Verification items for the finished model (mm, model axes). Coordinates: 2 decimals unless noted, no trailing zeros. Order: outer loops, then holes, each group sorted by start corner. A loop starts at its lowest first (then second) coordinate and runs counter-clockwise, first axis right, second up.
Q1. Cross-section at B-B, the plane z = 0. Record the boundary of the cut face in (x, y), and give its area (3 significant figures).
Q2. Cross-section at C-C, the plane y = -4.5. Count the separate pieces of the cut face and the enclosed holes in it, and give its area (3 significant figures).
Q3. Cross-section at D-D, the plane z = 36. Record the boundary of the cut face in (x, y).
Q4. Depth check by flat-ended pin: P1, Ø8.5, axis at x = 70.71, z = 70.71, coming from the -Y side; P2, Ø3.5, axis at x = -7.5, z = 0, coming from the +Y side; P3, Ø3, axis at y = -2.5, z = 75.5, coming from the -X side; P4, Ø2, axis at x = 6.5, y = -4.5, coming from the -Z side. Enter the tip coordinate at first touch or a pass-through.
Q5. Thickness scan on line 1 (X direction, y = -3.45, z = 0); line 2 (X direction, y = -2.65, z = 7.5); line 3 (Z direction, x = 69.5, y = -3.25). Record the ranges inside material, lowest first.
Q6. Cross-section at A-A, the plane x = 7.5. Record the boundary of the cut face in (y, z), and give its area (3 significant figures).
from build123d import *

# Parameters (mm, degrees)
SKETCH2_R                                       = 4.7625
SKETCH2_W                                       = 6.1
SKETCH2_H                                       = 6.1
BOSS_EXTRUDE1_DEPTH                             = 6.35
CSK_FOR_M3_FLAT_HEAD_MACHINE_SCREW1_D           = 3.2
CSK_FOR_M3_FLAT_HEAD_MACHINE_SCREW1_CSINK_D     = 6.3
CSK_FOR_M3_FLAT_HEAD_MACHINE_SCREW1_CSINK_ANGLE = 90


with BuildPart() as part:
    # Sketch2 → Boss-Extrude1 (new body)
    with BuildSketch(Plane(origin=(0, 0, 0), x_dir=(1, 0, 0), z_dir=(0, 1, 0))):
        with BuildLine():
            Line((10.606601718, 10.606601718), (81.317279836, -60.104076401))
            ThreePointArc((81.317279836, -60.104076401), (81.317279836, -81.317279836), (60.104076401, -81.317279836))
            Line((60.104076401, -81.317279836), (-10.606601718, -10.606601718))
            ThreePointArc((-10.606601718, -10.606601718), (-10.606601718, 10.606601718), (10.606601718, 10.606601718))
        make_face()
        with Locations(Location((70.710678119, -70.710678119, 0), (0, 0, 270))):
            Circle(SKETCH2_R, mode=Mode.SUBTRACT)
        Rectangle(SKETCH2_W, SKETCH2_H, mode=Mode.SUBTRACT)
    extrude(amount=-BOSS_EXTRUDE1_DEPTH)

    # CSK for M3 Flat Head Machine Screw1 (through all)
    with Locations(Plane(origin=(0, 0, -7.5), x_dir=(0, 0, 1), z_dir=(0, 1, 0))):
        with Locations((0, 0), (7.5, -7.5), (7.5, 7.5), (15, 0)):
            CounterSinkHole(CSK_FOR_M3_FLAT_HEAD_MACHINE_SCREW1_D / 2, CSK_FOR_M3_FLAT_HEAD_MACHINE_SCREW1_CSINK_D / 2, counter_sink_angle=CSK_FOR_M3_FLAT_HEAD_MACHINE_SCREW1_CSINK_ANGLE)


solid = part.part
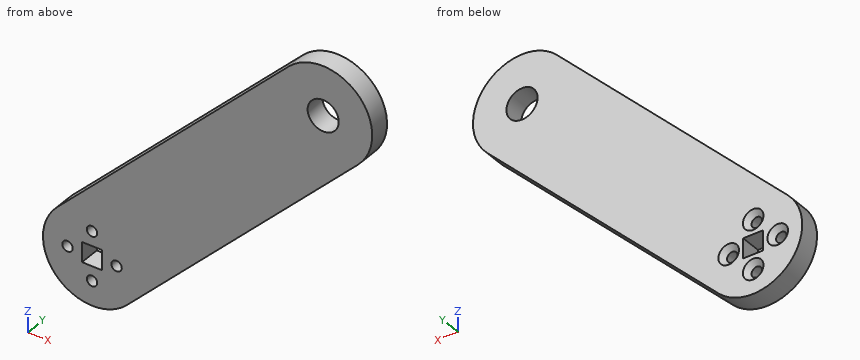
Check values:
1. outline: (-15, -6.35) - (-9.1, -6.35) - (-9.1, -1.55) - (-10.65, 0) - (-15, 0) - close; (-5.9, -6.35) - (-3.05, -6.35) - (-3.05, 0) - (-4.35, 0) - (-5.9, -1.55) - close; (3.05, -6.35) - (5.9, -6.35) - (5.9, -1.55) - (4.35, 0) - (3.05, 0) - close; (9.1, -6.35) - (21.21, -6.35) - (21.21, 0) - (10.65, 0) - (9.1, -1.55) - close
1. area: 146 mm2
2. separate pieces: 1
2. enclosed holes: 6
2. area: 3,570 mm2
3. outline: (14.79, -6.35) - (57.21, -6.35) - (57.21, 0) - (14.79, 0) - close
4. P1: passes through
4. P2: stops at y = -1.4
4. P3: stops at x = 52.79
4. P4: stops at z = -13.96
5. line 1: x = -15 to -9.1, -5.9 to -3.05, 3.05 to 5.9, 9.1 to 21.21
5. line 2: x = -12.99 to -1.6, 1.6 to 28.71
5. line 3: z = 48.29 to 66.1, 75.32 to 85.66
6. outline: (-6.35, -12.99) - (0, -12.99) - (0, -3.15) - (-1.55, -1.6) - (-6.35, -1.6) - close; (-6.35, 1.6) - (-1.55, 1.6) - (0, 3.15) - (0, 28.71) - (-6.35, 28.71) - close
6. area: 242 mm2
